The drawing under review shows one solid part. Ordinate dimensions are in mm from its lowest x, y, z. A direction names the side the tool comes from. Round coordinates to 2 decimals unless told otherwise and drop trailing zeros. Order: outer loops, then holes, each group sorted by start corner. A loop starts at its lowest first (then second) coordinate and runs counter-clockwise, first axis right, second up.
1) Consider section B-B (x = 788). Give the boundary of the cut face in (y, z), then the cut area to 3 significant figures.
2) Consider section C-C (z = 384). Give the boundary of the cut face in (x, y).
3) Consider section A-A (y = 227.5). Give the boundary of the cut face in (x, z), then the cut area to 3 significant figures.
4) To check wall thickness, follow L1, parallel to Z at x = 526, y = 152.5; L2, parallel to Y at x = 925.5, z = 641; L3, parallel to Z at x = 559.5, y = 36. State the ranges of each line that lie inside material, in increasing order.
5) Clearance check with flat-ended pins moving along their axes: P1, Ø12.5, axis at x = 456.5, z = 310.5, coming from the +Y side; P2, Ø14, axis at x = 365.5, y = 159, coming from the +Z side; P3, Ø12.5, axis at x = 603, z = 309.5, coming from the -Y side. State where each tip first meets the part, or that it passes through.
6) Consider section D-D (y = 408). Give the boundary of the cut face in (x, z).
7) Machinability: for the marked faces 1, 2 and 3, which of the approach directions +Z, -Z, +X, -X, +Y, -Y give a long, thin tool a straight path to every point of the face, cutting with its end or side? Answer none if there is none.
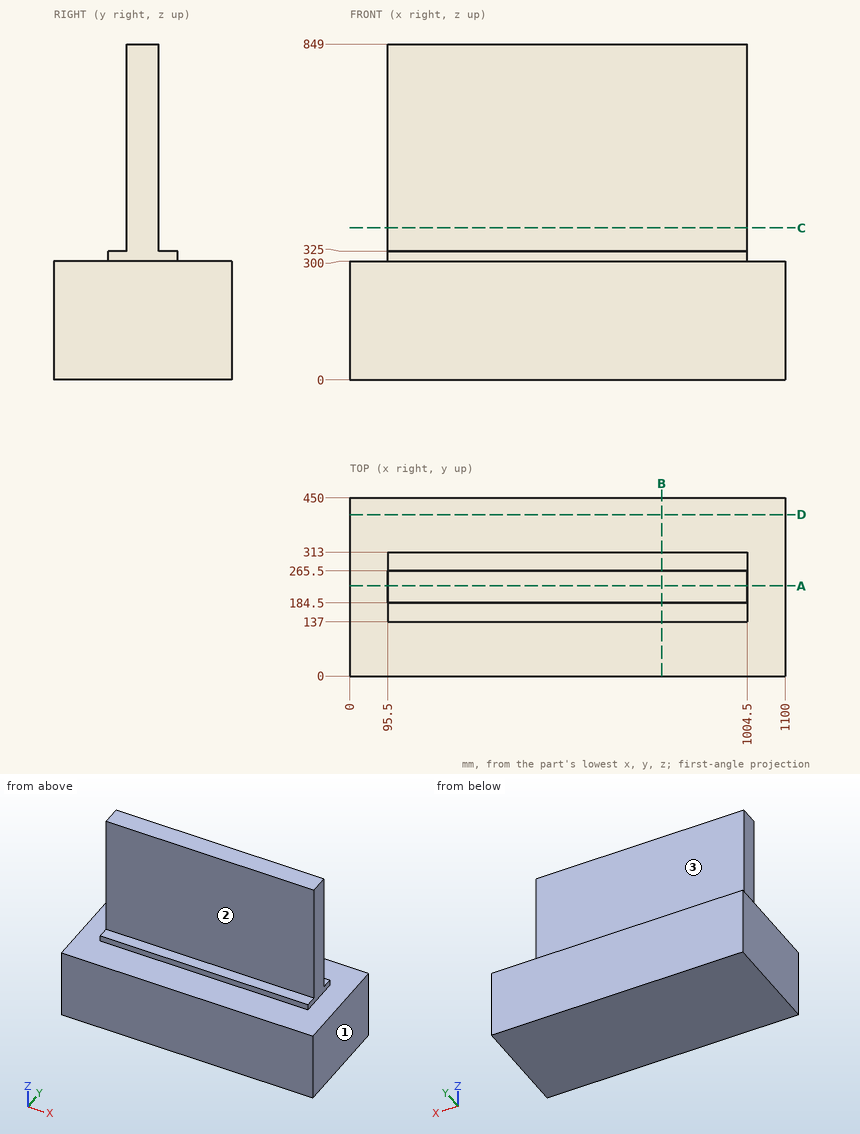
Answer below:
1. outline: (0, 0) - (450, 0) - (450, 300) - (313, 300) - (313, 325) - (265.5, 325) - (265.5, 849) - (184.5, 849) - (184.5, 325) - (137, 325) - (137, 300) - (0, 300) - close
1. area: 182,000 mm2
2. outline: (95.5, 184.5) - (1004.5, 184.5) - (1004.5, 265.5) - (95.5, 265.5) - close
3. outline: (0, 0) - (1100, 0) - (1100, 300) - (1004.5, 300) - (1004.5, 849) - (95.5, 849) - (95.5, 300) - (0, 300) - close
3. area: 829,000 mm2
4. L1: z = 0 to 325
4. L2: y = 184.5 to 265.5
4. L3: z = 0 to 300
5. P1: stops at y = 313
5. P2: stops at z = 325
5. P3: stops at y = 137
6. outline: (0, 0) - (1100, 0) - (1100, 300) - (0, 300) - close
7. face 1: +Z, -Z, +X, +Y, -Y
7. face 2: +Z, +X, -X, -Y
7. face 3: +Z, +X, -X, +Y
